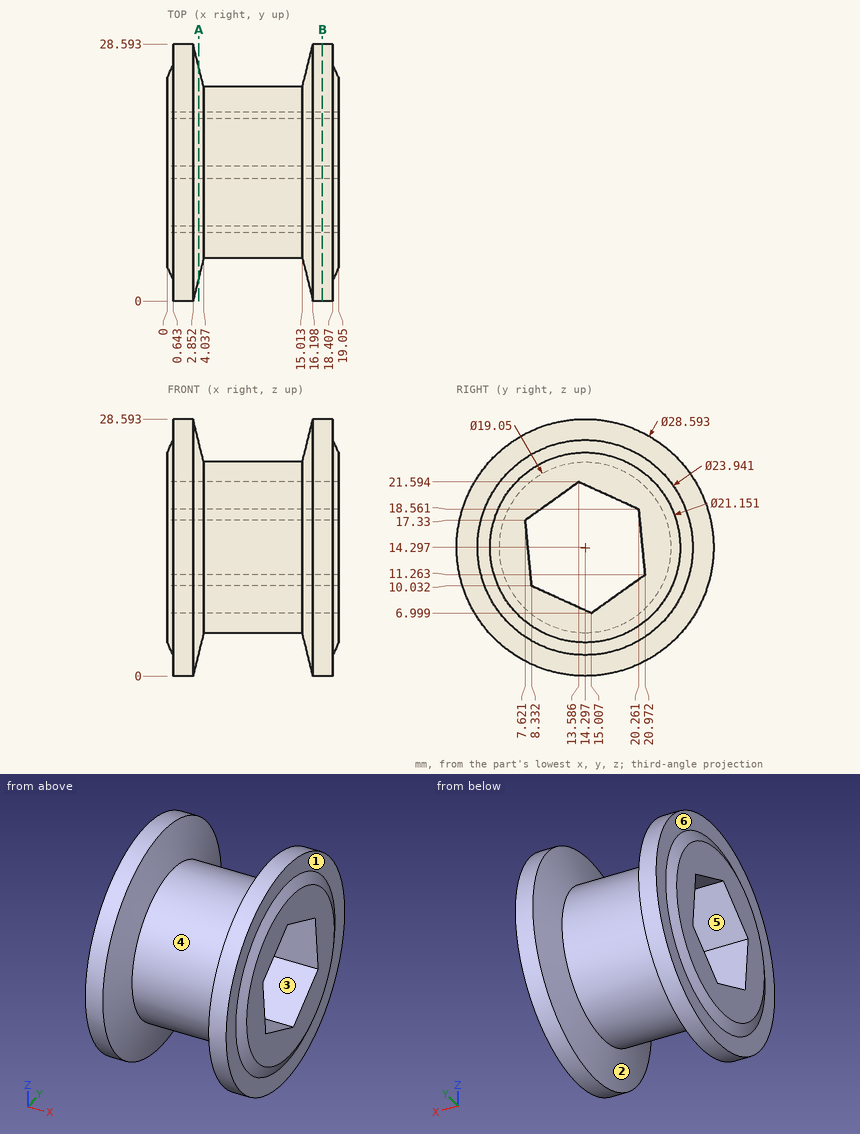
The drawing under review shows one solid part. Ordinate dimensions are in mm from its lowest x, y, z. A direction names the side the tool comes from. Give positions to 0.01 mm unless a question says otherwise; leave off trailing zeros. Write each loop counter-clockwise with the first axis right and the second up, starting at its lowest first coordinate (ties: lowest second). Pieces come first, ordered by that corner, then holes. Notation, with made-up numbers: (-8, 40.25) -> (33, 40.25) arc R11 cw to (33, 50.25) -> close; hole circle Ø4 at (-16, 60). An arc over 180 degrees is marked (long way). Put each result on its own line as item: value.
(1) Tool access review of the marked faces 4, 5 and 6: name each direction out of +Z, -Z, +X, -X, +Y, -Y from which nothing blocks a thin tool from reaching the whole face with its end or side.
Results are:
face 4: none
face 5: +X, -X
face 6: -X
(2) We need section A-A, the plane x = 3.5. Give the boundary of the cut face in (y, z) (1 decimal).
Results are:
outline: circle Ø23.4 at (14.3, 14.3); hole (7.6, 17.3) -> (8.3, 10) -> (15, 7) -> (21, 11.3) -> (20.3, 18.6) -> (13.6, 21.6) -> close
(3) To check wall thickness, follow probe 1 along Y at (x, z) = (11.5, 13.5) (1 decimal); probe 2 along X at (y, z) = (11, 5.25); probe 3 along Y at (x, z) = (5.25, 21.25) (1 decimal). State the ranges of each line that lie inside material, in increasing order. Write a range as from..to.
Results are:
probe 1: 4.8..8, 20.8..23.8
probe 2: 0..4.01, 15.04..19.05
probe 3: 7.8..13.1, 14.3..20.8
(4) We need section B-B, the plane x = 17.25. Give the boundary of the cut face in (y, z) (1 decimal).
Results are:
outline: circle Ø28.6 at (14.3, 14.3); hole (7.6, 17.3) -> (8.3, 10) -> (15, 7) -> (21, 11.3) -> (20.3, 18.6) -> (13.6, 21.6) -> close
(5) The part is to be moulded in two halves that separate along Y. For the marked faces 1, 2 and 3, say which applies: pulls with the +Y half, pulls with the -Y half, needs draft (parallel to the pull), parting line crosses it, or undercut.
Results are:
face 1: needs draft
face 2: parting line crosses it
face 3: undercut
(6) For pin 1 Ø10 at (x, z) = (11.5, 18.5) entering from +Y (1 decimal); pin 2 Ø6 at (y, z) = (5, 25.5) entering from +X; pin 3 Ø1 at (x, z) = (6.5, 13) entering from +Y, all flat-tipped, find the tip position at first contact; note any pin that passes through.
Results are:
pin 1: y = 28.4
pin 2: x = 18.6
pin 3: y = 23.79
